```python
from build123d import *

# Parameters (mm, degrees)
F0_W     = 487.68
F0_H     = 457.2
F1_DEPTH = 914.4
F3_DEPTH = 15.24
F5_W     = 15.24
F5_H     = 60.96
F6_DEPTH = 7.62
F8_DEPTH = 487.68
F9_R     = 15.24


with BuildPart() as f1:
    # F0 (on Top) → F1 (new body)
    with BuildSketch(Plane.XY):
        with Locations((-16.6927352548, 0.1030346877)):
            Rectangle(F0_W, F0_H)
    extrude(amount=F1_DEPTH)

    # F2 (on face) → F3 (join)
    with BuildSketch(Plane.XZ.offset(228.4969653123)):
        with BuildLine():
            ThreePointArc((-181.4615279436, 105.584), (-179.9970618495, 102.0484660941), (-176.4615279436, 100.584))
            Line((-176.4615279436, 100.584), (154.5883071423, 100.584))
            ThreePointArc((154.5883071423, 100.584), (158.1238410482, 102.0484660941), (159.5883071423, 105.584))
            Line((159.5883071423, 105.584), (159.5883071423, 808.816))
            ThreePointArc((159.5883071423, 808.816), (158.1238410482, 812.3515339059), (154.5883071423, 813.816))
            Line((154.5883071423, 813.816), (-176.4615279436, 813.816))
            ThreePointArc((-176.4615279436, 813.816), (-179.9970618495, 812.3515339059), (-181.4615279436, 808.816))
            Line((-181.4615279436, 808.816), (-181.4615279436, 105.584))
        make_face()
    extrude(amount=F3_DEPTH)

    # F4: F1 across face


with BuildPart() as f1_1:
    add(f1.part)
    add(f1.part.mirror(Plane(origin=(-16.6927352548, 0.1030346877, 0), x_dir=(1, 0, 0), z_dir=(0, 0, -1))))

    # F5 (on face) → F6 (join)
    with BuildSketch(Plane.XZ.offset(243.7369653123)):
        with Locations((130.6323071423, 630.936)):
            Rectangle(F5_W, F5_H)
        with Locations((130.6323071423, -283.464)):
            Rectangle(F5_W, F5_H)
    extrude(amount=F6_DEPTH)

    # F7 (on face) → F8 (cut)
    with BuildSketch(Plane.YZ.offset(227.1472647452)):
        Polygon((72.7191716433, 84.0164422989), (-228.4969653123, 84.0164422989), (-228.4969653123, -38.4914465249), (115.4544577003, -38.4914465249), align=None)
    extrude(amount=-F8_DEPTH, mode=Mode.SUBTRACT)

    # F9
    f9_edges = [f1_1.edges().sort_by_distance(p)[0] for p in [
        (-16.692735, -228.496965, -38.491447),
        (-16.692735, -228.496965, 84.016442),
    ]]
    fillet(f9_edges, radius=F9_R)


solid = f1_1.part
```
The listing builds one solid part. Answer for the finished solid, in the listing's coordinates (mm). A direction names the side the tool comes from. Give positions to 0.01 mm unless a question says otherwise; leave off trailing zeros. Order: outer loops, then holes, each group sorted by start corner. A loop starts at its lowest first (then second) coordinate and runs counter-clockwise, first axis right, second up.
Item 1: Which of the six approach directions +Z, -Z, +X, -X, +Y, -Y give full straight-line access (tool end or side, diameter ignored) to faces 1 (the face through (-13, -68, 84.016)), 2 (the face through (-20, 3, 914.4))?
From the geometry:
face 1: +X, -X, -Y
face 2: +Z, +X, -X, +Y, -Y
Item 2: Given pin 1 Ø8.5 at (y, z) = (-247, 618.5) entering from -X; pin 2 Ø2.5 at (x, y) = (127, -246.5) entering from +Z; pin 3 Ø4.5 at (y, z) = (-239.5, -417.5) entering from +X, each flat-ended and moving along its own axis, determine where each tip first touches the part or whether it passes through.
From the geometry:
pin 1: stops at x = -181.46
pin 2: stops at z = 661.42
pin 3: stops at x = 159.59
Item 3: Find the intervals of material crossed by probe 1 along Z at (x, y) = (-162.5, 35.5); probe 2 along Y at (x, z) = (-233, 809.5); probe 3 along Y at (x, z) = (4.5, 798.5), in increasing order.
From the geometry:
probe 1: z = -914.4 to -38.49, 84.02 to 914.4
probe 2: y = -228.5 to 228.7
probe 3: y = -243.74 to 228.7
Item 4: The part is cut by section D-D, the plane z = -284.5. Give the vertices of the cut face in (x, y).
From the geometry:
outline: (-260.53, -228.5) - (-181.46, -228.5) - (-181.46, -243.74) - (123.01, -243.74) - (123.01, -251.36) - (138.25, -251.36) - (138.25, -243.74) - (159.59, -243.74) - (159.59, -228.5) - (227.15, -228.5) - (227.15, 228.7) - (-260.53, 228.7) - close
Item 5: The part is cut by section A-A, the plane y = -32.5. Give the vertices of the cut face in (x, z), and give its area (3 significant figures).
From the geometry:
outline: (-260.53, -914.4) - (227.15, -914.4) - (227.15, -38.49) - (-260.53, -38.49) - close; (-260.53, 84.02) - (227.15, 84.02) - (227.15, 914.4) - (-260.53, 914.4) - close
area: 832,000 mm2
Item 6: For a pull along Z with two mould halves and no side action, classify faces 3 (the face through (-13.279, 94.386, 21.905)), 4 (the face through (-20, 3, -914.4)), 5 (the face through (-183, -228.497, -478)), 6 (the face through (-260.533, 99, 13)) as pulls with the +Z half, pulls with the -Z half, needs draft (parallel to the pull), parting line crosses it, or undercut.
From the geometry:
face 3: undercut
face 4: pulls with the -Z half
face 5: undercut
face 6: needs draft
Item 7: The part is cut by section C-C, the plane x = 83. Give the vertices of the cut face in (y, z), and give its area (3 significant figures).
From the geometry:
outline: (-243.74, -813.82) - (-228.5, -813.82) - (-228.5, -914.4) - (228.7, -914.4) - (228.7, 914.4) - (-228.5, 914.4) - (-228.5, 813.82) - (-243.74, 813.82) - (-243.74, 100.58) - (-228.5, 100.58) - (-228.5, 99.26) arc R15.24 ccw to (-213.26, 84.02) - (72.72, 84.02) - (115.45, -38.49) - (-213.26, -38.49) arc R15.24 ccw to (-228.5, -53.73) - (-228.5, -100.58) - (-243.74, -100.58) - close
area: 818,000 mm2
Item 8: The part is cut by section B-B, the plane z = 340. Give the vertices of the cut face in (x, y).
From the geometry:
outline: (-260.53, -228.5) - (-181.46, -228.5) - (-181.46, -243.74) - (159.59, -243.74) - (159.59, -228.5) - (227.15, -228.5) - (227.15, 228.7) - (-260.53, 228.7) - close
